Autodesk Inventor part; units mm, degrees
ref_plane "YZ Plane" through (0, 0, 0) normal (1, 0, 0) x (0, 1, 0)
ref_plane "XZ Plane" through (0, 0, 0) normal (0, 1, 0) x (-1, 0, 0)
ref_plane "XY Plane" through (0, 0, 0) normal (0, 0, 1) x (1, 0, 0)
sketch "Szkic1" plane through (0, 0, 0) normal (0, 1, 0) x (-1, 0, 0)
  line L0 (0, 0) -> (-100, 0)
  line L1 (-100, 0) -> (-100, -25)
  line L2 (-100, -25) -> (0, -25)
  line L3 (0, -25) -> (0, 0)
  dimension "d0" = 100
  dimension "d1" = 25
extrude "Wyciągnięcie proste1" add sketch "Szkic1" along normal blind 3
sketch "Szkic2" plane through (100, 0, 0) normal (1, 0, 0) x (0, 0, -1)
  line L0 (0, 0) -> (25, 0)
  line L1 (25, 0) -> (25, 3)
  line L2 (0, 3) -> (25, 3)
  line L3 (0, 0) -> (0, 3)
  line L4 (25, 0) -> (21.4247, 3)
  dimension "d4" = 40
extrude "Wyciągnięcie proste2" cut sketch "Szkic2" against normal through all contours L4 L2 L1
sketch "Szkic3" plane through (0, 0, 0) normal (0, -1, 0) x (1, 0, 0)
  line L0 (0, -25) -> (0, 0)
  line L1 (100, 0) -> (100, -25)
  line L2 (0, 0) -> (100, 0)
  line L3 (0, -25) -> (0, 0)
  line L4 (100, -25) -> (0, -25)
  point P0 (3.5, -3.5)
  dimension "d7" = 3.5
  dimension "d8" = 3.5
hole "Otwór1" at (3.5, 0, -3.5) direction (0, 1, 0) diameter 3.2 end through all countersink diameter 6 countersink angle 90
ref_plane "Płaszczyzna konstrukcyjna1" through (50, 0, 0) normal (-1, 0, 0) x (0, 0, 1)
mirror "Odbij1" about plane through (50, 0, 0) normal (-1, 0, 0) of "Otwór1"
properties part number "nóź" material "Stal, odlew"
Could you check a few things on this model? Use its own coordinates, in mm. Give positions to 0.01 mm unless a question says otherwise; leave off trailing zeros. Write each loop counter-clockwise with the first axis right and the second up, starting at its lowest first coordinate (ties: lowest second). Pieces come first, ordered by that corner, then holes. Notation, with made-up numbers: (64.25, -22.5) -> (93.25, -22.5) arc R26 ccw to (93.25, -1.5) -> close; hole circle Ø7 at (60, 28.5). An arc over 180 degrees is marked (long way). Write each question's results on one line, items separated by ' | '. Start each with the question number.
Q1. Suppose I cut it at C-C, the plane y = 0.85. List the corners of the cut face in (x, z) for me.
Q2. Suppose I cut it at B-B, the plane x = 96.5. List the corners of the cut face in (y, z) for me.
Q3. I need wall thicknesses on probe 1 along X at (y, z) = (2, -3.5); probe 2 along X at (y, z) = (1.7, -4); probe 3 along Z at (x, y) = (3.5, 2). Which ranges of each line are inside material? Lowest first, please.
Q4. We'd pull the mould along X, two halves only. Please class faces 1 (the face through (100, 1, -12)), 2 (the face through (51, 3, -11)), 3 (the face through (1.914, 2.211, -3.292)): +X half, -X half, draft (parallel to the pull), parting line (faces both ways), or undercut.
Q5. Suppose I cut it at A-A, the plane z = -3.5. List the corners of the cut face in (x, y) for me, and give its area (3 significant figures).
Q6. Suppose I cut it at D-D, the plane x = 58.5. List the corners of the cut face in (y, z) for me, and give its area (3 significant figures).
Q7. I'm going to push a flat-ended pin straight in: pin 1 Ø5 at (x, z) = (96.5, -3.5) entering from +Y. Where does the tip first touch, or does it pass through?
Outcome:
1) outline: (0, -23.99) -> (100, -23.99) -> (100, 0) -> (0, 0) -> close; hole circle Ø4.3 at (3.5, -3.5); hole circle Ø4.3 at (96.5, -3.5)
2) outline: (0, -25) -> (3, -21.42) -> (3, -5.1) -> (1.4, -5.1) -> (0, -6.5) -> close; (0, -0.5) -> (1.4, -1.9) -> (3, -1.9) -> (3, 0) -> (0, 0) -> close
3) probe 1: 0 to 1.9, 5.1 to 94.9, 98.1 to 100 | probe 2: 0 to 1.98, 5.02 to 94.98, 98.02 to 100 | probe 3: -22.62 to -5.1, -1.9 to 0
4) face 1: +X half | face 2: draft | face 3: undercut
5) outline: (0, 0) -> (0.5, 0) -> (1.9, 1.4) -> (1.9, 3) -> (0, 3) -> close; (5.1, 1.4) -> (6.5, 0) -> (93.5, 0) -> (94.9, 1.4) -> (94.9, 3) -> (5.1, 3) -> close; (98.1, 1.4) -> (99.5, 0) -> (100, 0) -> (100, 3) -> (98.1, 3) -> close | area: 277 mm2
6) outline: (0, -25) -> (3, -21.42) -> (3, 0) -> (0, 0) -> close | area: 69.6 mm2
7) pin 1: y = 3
